Read the model definition and answer for the solid it produces. Units are mm, in the model's axes. A direction names the side the tool comes from. Give positions to 0.01 mm unless a question says otherwise; leave off trailing zeros. Write each loop counter-clockwise with the first axis right and the second up, starting at its lowest first coordinate (ties: lowest second). Pieces come first, ordered by that corner, then holes.
```python
from build123d import *

# Parameters (mm, degrees)
CROQUIS1_R              = 3.25
CROQUIS1_R_2            = 2.5
SALIENTE_EXTRUIR1_DEPTH = 10
CROQUIS5_R              = 5.2
CORTAR_EXTRUIR2_DEPTH   = 5
FILLET1_R               = 3


with BuildPart() as part:
    # Croquis1 → Saliente-Extruir1 (new body)
    with BuildSketch(Plane(origin=(0, 0, 0), x_dir=(0, 0, -1), z_dir=(1, 0, 0))):
        Polygon((-25, -120), (25, -120), (25, 25), (0, 25), (-25, 25), (-25, 0), align=None)
        with Locations((-17.68, 17.68)):
            Circle(CROQUIS1_R, mode=Mode.SUBTRACT)
        with Locations(Location((17.68, 17.68, 0), (0, 0, 180))):
            Circle(CROQUIS1_R, mode=Mode.SUBTRACT)
        with Locations((17.68, -17.68)):
            Circle(CROQUIS1_R, mode=Mode.SUBTRACT)
        with Locations(Location((-17.68, -17.68, 0), (0, 0, 180))):
            Circle(CROQUIS1_R, mode=Mode.SUBTRACT)
        with Locations((-17.68, -114.5)):
            Circle(CROQUIS1_R_2, mode=Mode.SUBTRACT)
        with Locations(Location((17.68, -114.5, 0), (0, 0, 180))):
            Circle(CROQUIS1_R_2, mode=Mode.SUBTRACT)
    extrude(amount=SALIENTE_EXTRUIR1_DEPTH)

    # Croquis5 → Cortar-Extruir2 (cut)
    with BuildSketch(Plane(origin=(10, 0, 0), x_dir=(0, 0, -1), z_dir=(1, 0, 0))):
        with Locations((17.68, 17.68)):
            Circle(CROQUIS5_R)
        with Locations((-17.68, 17.68)):
            Circle(CROQUIS5_R)
        with Locations((-17.68, -17.68)):
            Circle(CROQUIS5_R)
        with Locations((17.68, -17.68)):
            Circle(CROQUIS5_R)
    extrude(amount=-CORTAR_EXTRUIR2_DEPTH, mode=Mode.SUBTRACT)

    # Fillet1
    fillet1_edges = [part.edges().sort_by_distance(p)[0] for p in [
        (5, 25, -25),
        (5, 25, 25),
    ]]
    fillet(fillet1_edges, radius=FILLET1_R)


solid = part.part
```
Item 1: Section A-A (y = -114.5) is taken. Write down the section's boundary in (x, z), and give its area (3 significant figures).
Result set:
outline: (0, -25) - (10, -25) - (10, -20.18) - (0, -20.18) - close; (0, -15.18) - (10, -15.18) - (10, 15.18) - (0, 15.18) - close; (0, 20.18) - (10, 20.18) - (10, 25) - (0, 25) - close
area: 400 mm2
Item 2: Determine the mould class of faces 3 (the cylindrical face through (5.07, 24.1, -24.14)), 4 (the cylindrical face through (7.54, -16.12, -22.64)), 5 (the cylindrical face through (2.465, -17.537, -14.433)), 6 (the flat face through (5, -48, 25)) for opening direction Z: pulls with the +Z half, pulls with the -Z half, needs draft (parallel to the pull), parting line crosses it, or undercut.
Result set:
face 3: pulls with the -Z half
face 4: undercut
face 5: undercut
face 6: pulls with the +Z half
Item 3: Which of the six approach directions +Z, -Z, +X, -X, +Y, -Y give full straight-line access (tool end or side, diameter ignored) to faces 1 (the cylindrical face through (4.93, -112.02, 18.01)), 2 (the flat face through (5, -15, 15))?
Result set:
face 1: +X, -X
face 2: +X
Item 4: Section B-B (z = -17.68) is taken. Write down the section's boundary in (x, y).
Result set:
outline: (0, -120) - (10, -120) - (10, -117) - (0, -117) - close; (0, -112) - (10, -112) - (10, -22.88) - (5, -22.88) - (5, -20.93) - (0, -20.93) - close; (0, -14.43) - (5, -14.43) - (5, -12.48) - (10, -12.48) - (10, 12.48) - (5, 12.48) - (5, 14.43) - (0, 14.43) - close; (0, 20.93) - (5, 20.93) - (5, 22.88) - (10, 22.88) - (10, 25) - (0, 25) - close
Item 5: Find the intervals of material crossed by line 1 along Y through (x, z) = (3, 17.5); line 2 along Y through (x, z) = (6.35, -17.68); line 3 along Z through (x, y) = (8.5, 14.5), in increasing order.
Result set:
line 1: y = -120 to -116.99, -112.01 to -20.93, -14.43 to 14.43, 20.93 to 25
line 2: y = -120 to -117, -112 to -22.88, -12.48 to 12.48, 22.88 to 25
line 3: z = -25 to -21.79, -13.57 to 13.57, 21.79 to 25
Item 6: Section D-D (y = 17.68) is taken. Write down the section's boundary in (x, z), and give its area (3 significant figures).
Result set:
outline: (0, -25) - (10, -25) - (10, -22.88) - (5, -22.88) - (5, -20.93) - (0, -20.93) - close; (0, -14.43) - (5, -14.43) - (5, -12.48) - (10, -12.48) - (10, 12.48) - (5, 12.48) - (5, 14.43) - (0, 14.43) - close; (0, 20.93) - (5, 20.93) - (5, 22.88) - (10, 22.88) - (10, 25) - (0, 25) - close
area: 331 mm2
Item 7: This flat-tipped pin is pushed along its axis until it touches: pin 1 Ø5 at (y, z) = (-19, 19.5) entering from +X. Where does it stop, or does it pass through?
Result set:
pin 1: stops at x = 5
Item 8: Section C-C (x = 6.75) is taken. Write down the section's boundary in (y, z), and give its area (3 significant figures).
Result set:
outline: (-120, -25) - (22, -25) arc R3 ccw to (25, -22) - (25, 22) arc R3 ccw to (22, 25) - (-120, 25) - close; hole circle Ø5 at (-114.5, -17.68); hole circle Ø5 at (-114.5, 17.68); hole circle Ø10.4 at (-17.68, -17.68); hole circle Ø10.4 at (-17.68, 17.68); hole circle Ø10.4 at (17.68, -17.68); hole circle Ø10.4 at (17.68, 17.68)
area: 6,870 mm2
